from build123d import *

# Parameters (mm, degrees)
EXTRUDE_1_DEPTH = 191


# Read off the part's stored shape, not the designer's step: 222 Конструкционный профиль 20х20-1-surface1
with BuildPart() as part:
    # Эскиз1 → Бобышка-Вытянуть1 (new body)
    with BuildSketch(Plane.XY):
        with BuildLine():
            Line((-3.945217202, 0.181521503), (-3.8, 0))
            Line((-3.8, 0), (-3.945217202, -0.181521503))
            ThreePointArc((-3.945217202, -0.181521503), (-3.98590708, -0.254943529), (-4, -0.337695265))
            Line((-4, -0.337695265), (-4, -1.898780669))
            ThreePointArc((-4, -1.898780669), (-4.152240935, -2.664147534), (-4.585786438, -3.312994231))
            Line((-4.585786438, -3.312994231), (-6.279898987, -5.007106781))
            ThreePointArc((-6.279898987, -5.007106781), (-6.604322336, -5.223879533), (-6.987005769, -5.3))
            Line((-6.987005769, -5.3), (-7.8, -5.3))
            ThreePointArc((-7.8, -5.3), (-7.941421356, -5.241421356), (-8, -5.1))
            Line((-8, -5.1), (-8, -3.33))
            ThreePointArc((-8, -3.33), (-8.154329142, -3.099030117), (-8.426776695, -3.153223305))
            Line((-8.426776695, -3.153223305), (-9.926776695, -4.653223305))
            ThreePointArc((-9.926776695, -4.653223305), (-9.980969883, -4.734329142), (-10, -4.83))
            Line((-10, -4.83), (-10, -8.5))
            ThreePointArc((-10, -8.5), (-9.560660172, -9.560660172), (-8.5, -10))
            Line((-8.5, -10), (-4.83, -10))
            ThreePointArc((-4.83, -10), (-4.734329142, -9.980969883), (-4.653223305, -9.926776695))
            Line((-4.653223305, -9.926776695), (-3.153223305, -8.426776695))
            ThreePointArc((-3.153223305, -8.426776695), (-3.099030117, -8.154329142), (-3.33, -8))
            Line((-3.33, -8), (-5.1, -8))
            ThreePointArc((-5.1, -8), (-5.241421356, -7.941421356), (-5.3, -7.8))
            Line((-5.3, -7.8), (-5.3, -6.987005769))
            ThreePointArc((-5.3, -6.987005769), (-5.223879533, -6.604322336), (-5.007106781, -6.279898987))
            Line((-5.007106781, -6.279898987), (-3.312994231, -4.585786438))
            ThreePointArc((-3.312994231, -4.585786438), (-2.664147534, -4.152240935), (-1.898780669, -4))
            Line((-1.898780669, -4), (-0.337695265, -4))
            ThreePointArc((-0.337695265, -4), (-0.254943529, -3.98590708), (-0.181521503, -3.945217202))
            Line((-0.181521503, -3.945217202), (0, -3.8))
            Line((0, -3.8), (0.181521503, -3.945217202))
            ThreePointArc((0.181521503, -3.945217202), (0.254943529, -3.98590708), (0.337695265, -4))
            Line((0.337695265, -4), (1.898780669, -4))
            ThreePointArc((1.898780669, -4), (2.664147534, -4.152240935), (3.312994231, -4.585786438))
            Line((3.312994231, -4.585786438), (5.007106781, -6.279898987))
            ThreePointArc((5.007106781, -6.279898987), (5.223879533, -6.604322336), (5.3, -6.987005769))
            Line((5.3, -6.987005769), (5.3, -7.8))
            ThreePointArc((5.3, -7.8), (5.241421356, -7.941421356), (5.1, -8))
            Line((5.1, -8), (3.33, -8))
            ThreePointArc((3.33, -8), (3.099030117, -8.154329142), (3.153223305, -8.426776695))
            Line((3.153223305, -8.426776695), (4.653223305, -9.926776695))
            ThreePointArc((4.653223305, -9.926776695), (4.734329142, -9.980969883), (4.83, -10))
            Line((4.83, -10), (8.5, -10))
            ThreePointArc((8.5, -10), (9.560660172, -9.560660172), (10, -8.5))
            Line((10, -8.5), (10, -4.83))
            ThreePointArc((10, -4.83), (9.980969883, -4.734329142), (9.926776695, -4.653223305))
            Line((9.926776695, -4.653223305), (8.426776695, -3.153223305))
            ThreePointArc((8.426776695, -3.153223305), (8.154329142, -3.099030117), (8, -3.33))
            Line((8, -3.33), (8, -5.1))
            ThreePointArc((8, -5.1), (7.941421356, -5.241421356), (7.8, -5.3))
            Line((7.8, -5.3), (6.987005769, -5.3))
            ThreePointArc((6.987005769, -5.3), (6.604322336, -5.223879533), (6.279898987, -5.007106781))
            Line((6.279898987, -5.007106781), (4.585786438, -3.312994231))
            ThreePointArc((4.585786438, -3.312994231), (4.152240935, -2.664147534), (4, -1.898780669))
            Line((4, -1.898780669), (4, -0.337695265))
            ThreePointArc((4, -0.337695265), (3.98590708, -0.254943529), (3.945217202, -0.181521503))
            Line((3.945217202, -0.181521503), (3.8, 0))
            Line((3.8, 0), (3.945217202, 0.181521503))
            ThreePointArc((3.945217202, 0.181521503), (3.98590708, 0.254943529), (4, 0.337695265))
            Line((4, 0.337695265), (4, 1.898780669))
            ThreePointArc((4, 1.898780669), (4.152240935, 2.664147534), (4.585786438, 3.312994231))
            Line((4.585786438, 3.312994231), (6.279898987, 5.007106781))
            ThreePointArc((6.279898987, 5.007106781), (6.604322336, 5.223879533), (6.987005769, 5.3))
            Line((6.987005769, 5.3), (7.8, 5.3))
            ThreePointArc((7.8, 5.3), (7.941421356, 5.241421356), (8, 5.1))
            Line((8, 5.1), (8, 3.33))
            ThreePointArc((8, 3.33), (8.154329142, 3.099030117), (8.426776695, 3.153223305))
            Line((8.426776695, 3.153223305), (9.926776695, 4.653223305))
            ThreePointArc((9.926776695, 4.653223305), (9.980969883, 4.734329142), (10, 4.83))
            Line((10, 4.83), (10, 8.5))
            ThreePointArc((10, 8.5), (9.560660172, 9.560660172), (8.5, 10))
            Line((8.5, 10), (4.83, 10))
            ThreePointArc((4.83, 10), (4.734329142, 9.980969883), (4.653223305, 9.926776695))
            Line((4.653223305, 9.926776695), (3.153223305, 8.426776695))
            ThreePointArc((3.153223305, 8.426776695), (3.099030117, 8.154329142), (3.33, 8))
            Line((3.33, 8), (5.1, 8))
            ThreePointArc((5.1, 8), (5.241421356, 7.941421356), (5.3, 7.8))
            Line((5.3, 7.8), (5.3, 6.987005769))
            ThreePointArc((5.3, 6.987005769), (5.223879533, 6.604322336), (5.007106781, 6.279898987))
            Line((5.007106781, 6.279898987), (3.312994231, 4.585786438))
            ThreePointArc((3.312994231, 4.585786438), (2.664147534, 4.152240935), (1.898780669, 4))
            Line((1.898780669, 4), (0.337695265, 4))
            ThreePointArc((0.337695265, 4), (0.254943529, 3.98590708), (0.181521503, 3.945217202))
            Line((0.181521503, 3.945217202), (0, 3.8))
            Line((0, 3.8), (-0.181521503, 3.945217202))
            ThreePointArc((-0.181521503, 3.945217202), (-0.254943529, 3.98590708), (-0.337695265, 4))
            Line((-0.337695265, 4), (-1.898780669, 4))
            ThreePointArc((-1.898780669, 4), (-2.664147534, 4.152240935), (-3.312994231, 4.585786438))
            Line((-3.312994231, 4.585786438), (-5.007106781, 6.279898987))
            ThreePointArc((-5.007106781, 6.279898987), (-5.223879533, 6.604322336), (-5.3, 6.987005769))
            Line((-5.3, 6.987005769), (-5.3, 7.8))
            ThreePointArc((-5.3, 7.8), (-5.241421356, 7.941421356), (-5.1, 8))
            Line((-5.1, 8), (-3.33, 8))
            ThreePointArc((-3.33, 8), (-3.099030117, 8.154329142), (-3.153223305, 8.426776695))
            Line((-3.153223305, 8.426776695), (-4.653223305, 9.926776695))
            ThreePointArc((-4.653223305, 9.926776695), (-4.734329142, 9.980969883), (-4.83, 10))
            Line((-4.83, 10), (-8.5, 10))
            ThreePointArc((-8.5, 10), (-9.560660172, 9.560660172), (-10, 8.5))
            Line((-10, 8.5), (-10, 4.83))
            ThreePointArc((-10, 4.83), (-9.980969883, 4.734329142), (-9.926776695, 4.653223305))
            Line((-9.926776695, 4.653223305), (-8.426776695, 3.153223305))
            ThreePointArc((-8.426776695, 3.153223305), (-8.154329142, 3.099030117), (-8, 3.33))
            Line((-8, 3.33), (-8, 5.1))
            ThreePointArc((-8, 5.1), (-7.941421356, 5.241421356), (-7.8, 5.3))
            Line((-7.8, 5.3), (-6.987005769, 5.3))
            ThreePointArc((-6.987005769, 5.3), (-6.604322336, 5.223879533), (-6.279898987, 5.007106781))
            Line((-6.279898987, 5.007106781), (-4.585786438, 3.312994231))
            ThreePointArc((-4.585786438, 3.312994231), (-4.152240935, 2.664147534), (-4, 1.898780669))
            Line((-4, 1.898780669), (-4, 0.337695265))
            ThreePointArc((-4, 0.337695265), (-3.98590708, 0.254943529), (-3.945217202, 0.181521503))
        make_face()
    extrude(amount=EXTRUDE_1_DEPTH)


solid = part.part
Source: CAD feature listing. Evaluate the final solid. Frame: model axes, mm. Give positions to 0.01 mm unless a question says otherwise; leave off trailing zeros. Use a Markdown table: item, result.
1) Contact query for flat-ended pins moving along their axis: P1, Ø1.4, axis at x = 4, z = 85, coming from the -Y side; P2, Ø0.5, axis at y = -1.5, z = 115.5, coming from the +X side; P3, Ø2, axis at x = 3, z = 47, coming from the +Y side. Output: stop coordinate, or through.
Answer list:
| item | result |
|---|---|
| P1 | y = -9.96 |
| P2 | x = 4 |
| P3 | y = 9.27 |
2) Mould query, pull axis Y, two halves, no side actions, for faces 1 (the flat face through (0, 0, 191)), 2 (the flat face through (-7, -10, 94)), 3 (the flat face through (-7, 10, 94)). Classes: +Y half, -Y half, draft (parallel to the pull), parting line (faces both ways), or undercut.
Answer list:
| item | result |
|---|---|
| face 1 | draft |
| face 2 | -Y half |
| face 3 | +Y half |
3) Ray query, line 1 along Y through (x, z) = (-7.5, 118.5); line 2 along X through (y, z) = (8.25, 64). Return the intervals inside material, ascending. Write a range as [from, to].
Answer list:
| item | result |
|---|---|
| line 1 | [-10, -5.3], [5.3, 10] |
| line 2 | [-10, -3.08], [3.08, 10] |
